Input: dimensioned drawing with shaded views. Units: mm. Origin: part minimum x, y, z. A direction names the side the tool comes from. Give positions to 0.01 mm unless a question says otherwise; leave off trailing zeros. Loops run counter-clockwise (first coordinate to the right, second up) from the corner with the lowest first, then second, coordinate; pieces in that order, holes last. Notation, with made-up numbers: M 58,29.25 L 96,29.25 A10 cw 96,45.25 Z; hole C 78.5,54 d2. An arc over 180 degrees is marked long. Answer in a Markdown table with one row per item.
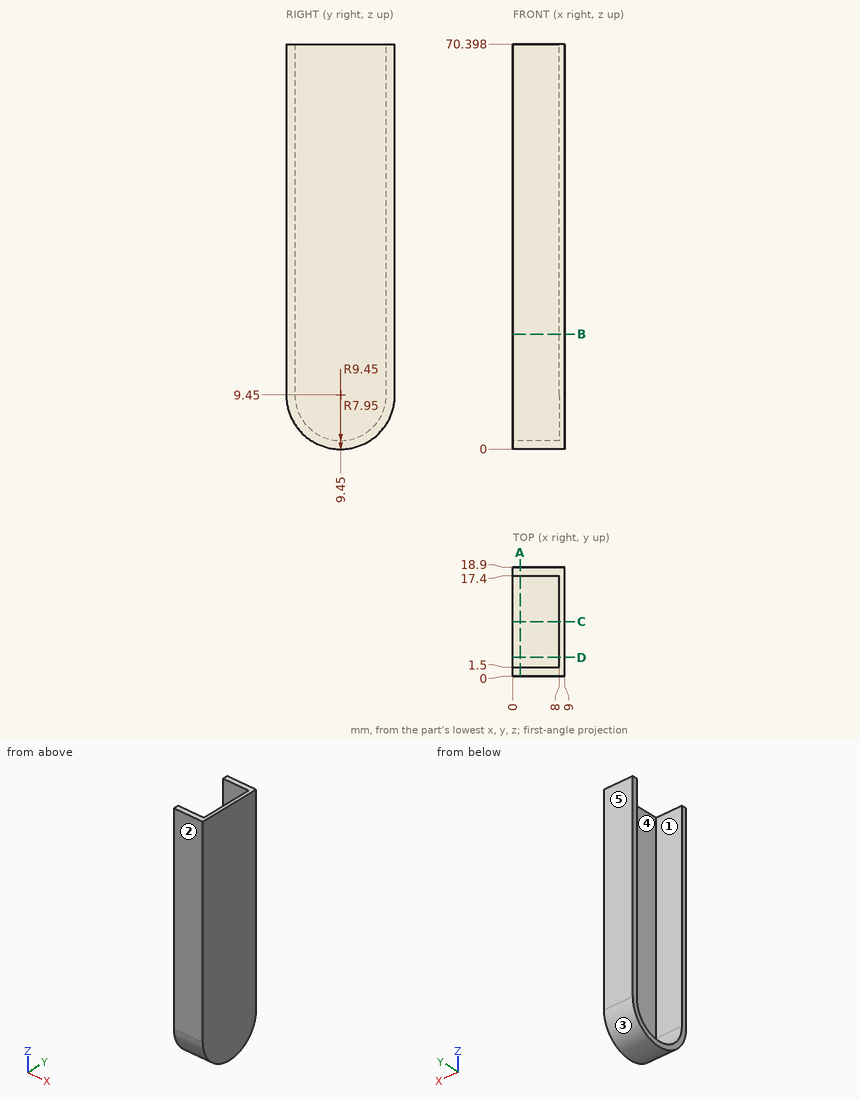
Q1. Contact query for a flat-ended pin moving along its axis: pin 1 Ø10 at (y, z) = (9.5, 42) entering from -X. Output: stop coordinate, or through.
Values follow:
| item | result |
|---|---|
| pin 1 | x = 8 |
Q2. Mould query, pull axis Y, two halves, no side actions, for the marked faces 3, 4 and 5. Classes: +Y half, -Y half, draft (parallel to the pull), parting line (faces both ways), or undercut.
Values follow:
| item | result |
|---|---|
| face 3 | parting line |
| face 4 | undercut |
| face 5 | +Y half |
Q3. Ray query, probe 1 along Y at (x, z) = (5.75, 51); probe 2 along X at (y, z) = (15.25, 56.5); probe 3 along Z at (x, y) = (8.25, 16.5). Return the intervals inside material, ascending. Write a range as from..to.
Values follow:
| item | result |
|---|---|
| probe 1 | 0..1.5, 17.4..18.9 |
| probe 2 | 8..9 |
| probe 3 | 3.16..70.4 |
Q4. Section query B-B (z = 20). Output: boundary loops of the cut face in (x, y).
Values follow:
| item | result |
|---|---|
| outline | M 0,0 L 9,0 L 9,18.9 L 0,18.9 L 0,17.4 L 8,17.4 L 8,1.5 L 0,1.5 Z |
Q5. Section query C-C (y = 9.45). Output: boundary loops of the cut face in (x, z).
Values follow:
| item | result |
|---|---|
| outline | M 0,0 L 9,0 L 9,70.4 L 8,70.4 L 8,1.5 L 0,1.5 Z |
Q6. Reachability of the marked faces 1 and 2 from +Z, -Z, +X, -X, +Y, -Y: full face, straight path, thin tool, end or side. Return the list, or none.
Values follow:
| item | result |
|---|---|
| face 1 | +Z, -X |
| face 2 | +Z, -Z, +X, -X, -Y |
Q7. Section query A-A (x = 1.25). Output: boundary loops of the cut face in (y, z).
Values follow:
| item | result |
|---|---|
| outline | M 0,9.45 A9.45 ccw 18.9,9.45 L 18.9,70.4 L 17.4,70.4 L 17.4,9.45 A7.95 cw 1.5,9.45 L 1.5,70.4 L 0,70.4 Z |
Q8. Section query D-D (y = 3.25). Output: boundary loops of the cut face in (x, z).
Values follow:
| item | result |
|---|---|
| outline | M 0,2.32 L 9,2.32 L 9,70.4 L 8,70.4 L 8,4.47 L 0,4.47 Z |
